Work out the finished part from the listing and answer in its coordinate system (mm). A direction names the side the tool comes from. Round coordinates to 2 decimals unless told otherwise and drop trailing zeros. Loops run counter-clockwise (first coordinate to the right, second up) from the corner with the lowest first, then second, coordinate; pieces in that order, holes last. Notation, with made-up numbers: (33.25, -15.75) - (85.25, -15.75) arc R32 ccw to (85.25, 16.25) - close; hole circle Ø7 at (7.25, 1). An arc over 180 degrees is marked (long way). Answer as CSV lines item,"result". Start each with the question number.
Q1. For faces 1 (the face through (1.83, 20.7, -9.15)), 2 (the face through (5, -15.875, -4)), 3 (the face through (5, -19, 0)), determine the directions among +Z, -Z, +X, -X, +Y, -Y from which every point of the face is accessible in a straight line to the end or side of a thin tool.
Q2. Straight lines are drawn through the part: L1, parallel to X at y = -19.05, z = -1.65 (3 decimals); L2, parallel to Z at x = 6, y = 19.5; L3, parallel to Y at x = 6.25, z = -1.5 (3 decimals). For each, find the intervals that lie inside material, in ascending order. Write a range as [from, to].
Q3. Section A-A on x = 6.75 is taken. Count the separate pieces of the cut face and the enclosed holes in it, then the cut area to 3 significant figures.
Q4. Section C-C on z = 13.5 is taken. Write down the section's boundary in (x, y) (3 decimals).
Q5. Each of these flat-tipped pins is pushed along its axis until it touches: pin 1 Ø1 at (x, z) = (5, 11) entering from +Y; pin 2 Ø2 at (x, y) = (1.5, 10) entering from -Z; pin 3 Ø4 at (x, y) = (4, 12) entering from -Z; pin 4 Ø1.6 at (y, z) = (20.64, 0) entering from +X. Where does it stop, or does it pass through?
Q6. The mould has two halves that part along Z. Classify faces 4 (the face through (9.525, 0, 19)), 5 (the face through (4.696, 21.887, -0.518)): +Z half, -Z half, draft (parallel to the pull), parting line (faces both ways), or undercut.
```python
from build123d import *

# Parameters (mm, degrees)
F0_R     = 1.35255
F1_DEPTH = 9.525
F2_R     = 3.175
F3_DEPTH = 50.8
F4_R     = 1.190625
F5_DEPTH = 6.35


# Not quite as in the source:
# - a feature names something its author has since deleted; it is built from what else it names


with BuildPart() as f1:
    # F0 (on Right) → F1 (new body)
    with BuildSketch(Plane.YZ):
        with BuildLine():
            Line((-15.875, -12.7), (-15.875, 0))
            ThreePointArc((-15.875, 0), (-11.2253201513, 11.2253201513), (0, 15.875))
            ThreePointArc((0, 15.875), (11.2253201513, 11.2253201513), (15.875, 0))
            Line((15.875, 0), (15.875, -12.7))
            Line((15.875, -12.7), (25.4, -12.7))
            Line((25.4, -12.7), (25.4, 0))
            Line((25.4, 0), (25.4, 3.175))
            ThreePointArc((25.4, 3.175), (17.9605122421, 21.1355122421), (0, 28.575))
            ThreePointArc((0, 28.575), (-17.9605122421, 21.1355122421), (-25.4, 3.175))
            Line((-25.4, 3.175), (-25.4, 0))
            Line((-25.4, 0), (-25.4, -12.7))
            Line((-25.4, -12.7), (-15.875, -12.7))
        make_face()
        with Locations((20.6375, 0)):
            Circle(F0_R, mode=Mode.SUBTRACT)
    extrude(amount=F1_DEPTH)

    # F2 (on face) → F3 (cut)
    with BuildSketch(Plane(origin=(0, 25.4, 0), x_dir=(-1, 0, 0), z_dir=(0, 1, 0))):
        with Locations((-4.7625, -7.9375)):
            Circle(F2_R)
        with BuildLine():
            ThreePointArc((-4.7625, -12.7), (-8.1300960454, -11.3050960454), (-9.525, -7.9375))
            Line((-9.525, -7.9375), (-9.525, -12.7))
            Line((-9.525, -12.7), (-4.7625, -12.7))
        make_face()
        with BuildLine():
            ThreePointArc((0, -7.9375), (-1.3949039546, -11.3050960454), (-4.7625, -12.7))
            Line((-4.7625, -12.7), (0, -12.7))
            Line((0, -12.7), (0, -7.9375))
        make_face()
    extrude(amount=-F3_DEPTH, mode=Mode.SUBTRACT)

    # F4 (on Top) → F5 (cut)
    with BuildSketch(Plane.XY):
        with Locations((4.7625, -19.05)):
            Circle(F4_R)
    extrude(amount=-F5_DEPTH, mode=Mode.SUBTRACT)


solid = f1.part
```
Findings:
1,face 1,"+Y, -Y"
1,face 2,"-Z, +X, -X"
1,face 3,"none"
2,L1,"x = [0, 3.572], [5.953, 9.525]"
2,L2,"z = [-12.54, -10.86], [-5.01, -0.73], [0.73, 19.45]"
2,L3,"y = [-25.4, -15.875], [15.875, 25.4]"
3,separate pieces,"3"
3,enclosed holes,"1"
3,area,"912 mm^2"
4,outline,"(0, -23.207) - (9.525, -23.207) - (9.525, -8.353) - (0, -8.353) - close; (0, 8.353) - (9.525, 8.353) - (9.525, 23.207) - (0, 23.207) - close"
5,pin 1,"stops at y = 24.32"
5,pin 2,"stops at z = 11.45"
5,pin 3,"stops at z = 7.48"
5,pin 4,"passes through"
6,face 4,"draft"
6,face 5,"undercut"
